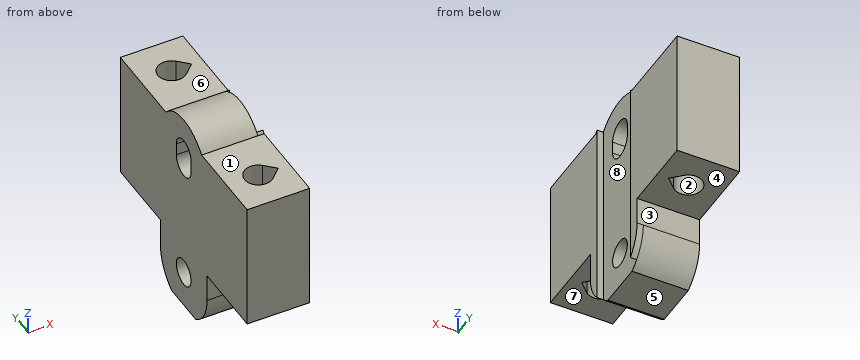
from build123d import *

# Parameters (mm, degrees)
BOSS_EXTRUDE1_DEPTH = 9
BOSS_EXTRUDE2_DEPTH = 1
BOSS_EXTRUDE3_DEPTH = 1
SKETCH4_W           = 10
SKETCH4_H           = 21
BOSS_EXTRUDE4_DEPTH = 12
SKETCH5_W           = 10
SKETCH5_H           = 21
BOSS_EXTRUDE5_DEPTH = 12
CUT_EXTRUDE1_DEPTH  = 34.693619574
CUT_EXTRUDE2_DEPTH  = 28.699277969
CUT_EXTRUDE3_DEPTH  = 34.693619574
HOLE1_D             = 4.4


with BuildPart() as part:
    # Sketch1 → Boss-Extrude1 (new body)
    with BuildSketch(Plane(origin=(4.9, 0, 0), x_dir=(0, -1, 0), z_dir=(-1, 0, 0))):
        with BuildLine():
            Line((7, -10.5), (7, 15))
            Line((7, 15), (5.361902647, 15))
            ThreePointArc((5.361902647, 15), (0, 17.5), (-5.361902647, 15))
            Line((-5.361902647, 15), (-7, 15))
            Line((-7, 15), (-7, -10.5))
            ThreePointArc((-7, -10.5), (-6.092571663, -13.946820352), (-3.605551275, -16.5))
            Line((-3.605551275, -16.5), (3.605551275, -16.5))
            ThreePointArc((3.605551275, -16.5), (6.092571663, -13.946820352), (7, -10.5))
        make_face()
    extrude(amount=-BOSS_EXTRUDE1_DEPTH)

    # Sketch2 → Boss-Extrude2 (add)
    with BuildSketch(Plane(origin=(13.9, 0, 0), x_dir=(0, 0, -1), z_dir=(1, 0, 0))):
        with BuildLine():
            Line((-15, -7), (-15, -5.361902647))
            ThreePointArc((-15, -5.361902647), (-15.202979206, -5.184784141), (-15.398993058, -4.999986702))
            Line((-15.398993058, -4.999986702), (15.398993058, -4.999986702))
            ThreePointArc((15.398993058, -4.999986702), (13.145760107, -6.480737107), (10.5, -7))
            Line((10.5, -7), (-15, -7))
        make_face()
    extrude(amount=BOSS_EXTRUDE2_DEPTH)

    # Sketch3 → Boss-Extrude3 (add)
    with BuildSketch(Plane(origin=(13.9, 0, 0), x_dir=(0, 0, -1), z_dir=(1, 0, 0))):
        with BuildLine():
            Line((-15, 7), (10.5, 7))
            ThreePointArc((10.5, 7), (13.145742515, 6.480744289), (15.398965913, 5.000013298))
            Line((15.398965913, 5.000013298), (-15.398965913, 5.000013298))
            ThreePointArc((-15.398965913, 5.000013298), (-15.202965132, 5.184796907), (-15, 5.361902647))
            Line((-15, 5.361902647), (-15, 7))
        make_face()
    extrude(amount=BOSS_EXTRUDE3_DEPTH)

    # Sketch4 → Boss-Extrude4 (add)
    with BuildSketch(Plane.XZ.offset(7)):
        with Locations((9.9, 4.5)):
            Rectangle(SKETCH4_W, SKETCH4_H)
    extrude(amount=BOSS_EXTRUDE4_DEPTH)

    # Sketch5 → Boss-Extrude5 (add)
    with BuildSketch(Plane(origin=(0, 7, 0), x_dir=(-1, 0, 0), z_dir=(0, 1, 0))):
        with Locations((-9.9, 4.5)):
            Rectangle(SKETCH5_W, SKETCH5_H)
    extrude(amount=BOSS_EXTRUDE5_DEPTH)

    # Sketch6 → Cut-Extrude1 (cut, through all)
    with BuildSketch(Plane(origin=(0, 0, -6), x_dir=(-1, 0, 0), z_dir=(0, 0, -1))):
        with BuildLine():
            Line((-11.428248415, 14.582547561), (-13.067024387, 13))
            Line((-13.067024387, 13), (-11.428248415, 11.417452439))
            ThreePointArc((-11.428248415, 11.417452439), (-7.7, 13), (-11.428248415, 14.582547561))
        make_face()
    extrude(amount=-CUT_EXTRUDE1_DEPTH, mode=Mode.SUBTRACT)

    # Sketch7 → Cut-Extrude2 (cut, through all)
    with BuildSketch(Plane.ZY.offset(-4.9)):
        with BuildLine():
            Line((9.5, -2.2), (11.5, -2.2))
            ThreePointArc((11.5, -2.2), (13.7, 0), (11.5, 2.2))
            Line((11.5, 2.2), (9.5, 2.2))
            ThreePointArc((9.5, 2.2), (7.3, 0), (9.5, -2.2))
        make_face()
    extrude(amount=-CUT_EXTRUDE2_DEPTH, mode=Mode.SUBTRACT)

    # Sketch8 → Cut-Extrude3 (cut, through all)
    with BuildSketch(Plane(origin=(0, 0, -6), x_dir=(-1, 0, 0), z_dir=(0, 0, -1))):
        with BuildLine():
            Line((-11.428248415, -11.417452439), (-13.067024387, -13))
            Line((-13.067024387, -13), (-11.428248415, -14.582547561))
            ThreePointArc((-11.428248415, -14.582547561), (-7.7, -13), (-11.428248415, -11.417452439))
        make_face()
    extrude(amount=-CUT_EXTRUDE3_DEPTH, mode=Mode.SUBTRACT)

    # Hole1 (through all)
    with Locations(Plane(origin=(13.9, 0, 0), x_dir=(0, 0, -1), z_dir=(1, 0, 0))):
        with Locations((10.5, 0)):
            Hole(HOLE1_D / 2)


solid = part.part
Check sheet for the modelled part. Datum: model origin and axes. Units: mm. Face numbers are marked on the shaded views. A direction names the side the tool comes from. Round coordinates to 2 decimals unless told otherwise and drop trailing zeros. Loops run counter-clockwise (first coordinate to the right, second up) from the corner with the lowest first, then second, coordinate; pieces in that order, holes last.
1. Set-up check for the marked faces 4, 5, 6, 7 and 8: record each of +Z, -Z, +X, -X, +Y, -Y from which the full face is reachable in a straight line by a thin tool's end or side.
2. Scan lines: probe 1 along Y at (x, z) = (9.9, 10.75); probe 2 along Y at (x, z) = (9.9, 3.25); probe 3 along Y at (x, z) = (10.5, -2). Record each from-to range of solid material in increasing order.
3. Gauge pin test, flat ends, axial feed: pin 1 Ø2 at (x, y) = (9.5, -8.5) entering from -Z; pin 2 Ø1 at (x, y) = (11.5, 1) entering from +Z; pin 3 Ø5 at (x, y) = (12.5, 10) entering from +Z. Record the tip position at first contact, or that the pin passes through.
4. Mould release check, pull along Y, two halves, no side actions. Record for the marked faces 1, 2 and 3: released by +Y, released by -Y, zero draft, split by the parting line, or undercut.
5. Sectioned sample at A-A on x = 9.9. Record the boundary of the cut face in (y, z), and give its area (3 significant figures).
6. Sectioned sample at B-B on y = 0. Record the boundary of the cut face in (x, z).
7. Sectioned sample at D-D on x = 12.5. Record the boundary of the cut face in (y, z), and give its area (3 significant figures).
8. Sectioned sample at C-C on z = 6.5. Record the boundary of the cut face in (x, y), and give its area (3 significant figures).
Recorded:
1. face 4: -Z, +X, -X, +Y
1. face 5: -Z, +X, -X, +Y, -Y
1. face 6: +Z, +X, -X, +Y
1. face 7: -Z, +X, -X, -Y
1. face 8: +Z, -Z, +X
2. probe 1: y = -19 to -15.2, -10.8 to -2.2, 2.2 to 10.8, 15.2 to 19
2. probe 2: y = -19 to -15.2, -10.8 to 10.8, 15.2 to 19
2. probe 3: y = -19 to -15.12, -10.88 to 10.88, 15.12 to 19
3. pin 1: stops at z = -6
3. pin 2: stops at z = 17.48
3. pin 3: stops at z = 15
4. face 1: zero draft
4. face 2: undercut
4. face 3: released by +Y
5. outline: (-19, -6) - (-15.2, -6) - (-15.2, 15) - (-19, 15) - close; (-10.8, -6) - (-7, -6) - (-7, -10.5) arc R7 ccw to (-3.61, -16.5) - (3.61, -16.5) arc R7 ccw to (7, -10.5) - (7, -6) - (10.8, -6) - (10.8, 15) - (5.36, 15) arc R7 ccw to (-5.36, 15) - (-10.8, 15) - close; (15.2, -6) - (19, -6) - (19, 15) - (15.2, 15) - close; hole circle Ø4.4 at (0, -10.5); hole (-2.2, 9.5) arc R2.2 ccw to (2.2, 9.5) - (2.2, 11.5) arc R2.2 ccw to (-2.2, 11.5) - close
5. area: 728 mm2
6. outline: (4.9, -16.5) - (13.9, -16.5) - (13.9, -12.7) - (4.9, -12.7) - close; (4.9, -8.3) - (13.9, -8.3) - (13.9, 7.3) - (4.9, 7.3) - close; (4.9, 13.7) - (13.9, 13.7) - (13.9, 17.5) - (4.9, 17.5) - close
7. outline: (-19, -6) - (-13.55, -6) - (-13.55, 15) - (-19, 15) - close; (-12.45, -6) - (-7, -6) - (-7, -10.5) arc R7 ccw to (-3.61, -16.5) - (3.61, -16.5) arc R7 ccw to (7, -10.5) - (7, -6) - (12.45, -6) - (12.45, 15) - (5.36, 15) arc R7 ccw to (-5.36, 15) - (-12.45, 15) - close; (13.55, -6) - (19, -6) - (19, 15) - (13.55, 15) - close; hole circle Ø4.4 at (0, -10.5); hole (-2.2, 9.5) arc R2.2 ccw to (2.2, 9.5) - (2.2, 11.5) arc R2.2 ccw to (-2.2, 11.5) - close
7. area: 867 mm2
8. outline: (4.9, -19) - (14.9, -19) - (14.9, -5) - (13.9, -5) - (13.9, 5) - (14.9, 5) - (14.9, 19) - (4.9, 19) - close; hole (11.43, -14.58) - (13.07, -13) - (11.43, -11.42) arc R2.2 ccw (long way) to start; hole (11.43, 11.42) - (13.07, 13) - (11.43, 14.58) arc R2.2 ccw (long way) to start
8. area: 337 mm2
